Read the model definition and answer for the solid it produces. Units are mm, in the model's axes. A direction names the side the tool comes from. Coordinates: 2 decimals unless noted, no trailing zeros. Loops run counter-clockwise (first coordinate to the right, second up) from the corner with the lowest first, then second, coordinate; pieces in that order, holes last. Notation, with made-up numbers: (14.25, -39) -> (62.25, -39) arc R21 cw to (62.25, -6) -> close; hole circle Ø6 at (-21, 35). An arc over 180 degrees is marked (long way). Answer in a Markdown table with one row per item.
```python
from build123d import *

# Parameters (mm, degrees)
EXTRUSION1_DEPTH        = 5
ESQUISSE2_R             = 1.5
EXTRUSION2_DEPTH        = 3
CHANFREIN1_SIZE         = 0.2
ESQUISSE3_R             = 1.3
ENL_V_MAT_EXTRU_1_DEPTH = 3


with BuildPart() as part:
    # Esquisse1 → Extrusion1 (new body)
    with BuildSketch(Plane.XY):
        Polygon((1.443375673, 2.5), (-1.443375673, 2.5), (-2.886751346, 0), (-1.443375673, -2.5), (1.443375673, -2.5), (2.886751346, 0), align=None)
    extrude(amount=EXTRUSION1_DEPTH)

    # Esquisse2 → Extrusion2 (add)
    with BuildSketch(Plane(origin=(0, 0, 0), x_dir=(-1, 0, 0), z_dir=(0, 0, -1))):
        Circle(ESQUISSE2_R)
    extrude(amount=EXTRUSION2_DEPTH)

    # Chanfrein1
    chanfrein1_edges = [part.edges().sort_by_distance(p)[0] for p in [
        (1.5, 0, -3),
    ]]
    chamfer(chanfrein1_edges, length=CHANFREIN1_SIZE)

    # Esquisse3 → Enlèv. mat.-Extru.1 (cut)
    with BuildSketch(Plane.XY.offset(5)):
        Circle(ESQUISSE3_R)
    extrude(amount=-ENL_V_MAT_EXTRU_1_DEPTH, mode=Mode.SUBTRACT)

    # Esquisse4 → Enlèvement de matière-Révolution1 (revolve, cut)
    with BuildSketch(Plane(origin=(0, 0, 0), x_dir=(1, 0, 0), z_dir=(0, 1, 0)), mode=Mode.PRIVATE) as enl_vement_de_mati_re_r_volution1_sk:
        with BuildLine():
            Line((1.2, 0.617157288), (1.2, 0.2))
            ThreePointArc((1.2, 0.2), (1.258578644, 0.058578644), (1.4, 0))
            Line((1.4, 0), (1.804772915, 0))
            Line((1.804772915, 0), (1.804772915, 1.304772915))
            Line((1.804772915, 1.304772915), (1.258578644, 0.758578644))
            ThreePointArc((1.258578644, 0.758578644), (1.215224093, 0.693693974), (1.2, 0.617157288))
        make_face()
    revolve(enl_vement_de_mati_re_r_volution1_sk.sketch.rotate(Axis((0, 0, -4.374841009), (0, 0, 1)), 180), axis=Axis((0, 0, -4.374841009), (0, 0, 1)), mode=Mode.SUBTRACT)


solid = part.part
```
1. A cutting plane is placed at D-D on x = -1.95. Give the vertices of the cut face in (y, z).
A:
| item | result |
|---|---|
| outline | (-1.62, 0) -> (1.62, 0) -> (1.62, 5) -> (-1.62, 5) -> close |
2. A tool of negligible diameter and unlimited length cuts with its end or side. For faces 5 (the cylindrical face through (1.5, 0.07, -1.89)), 6 (the flat face through (2.175, 1.233, 2.465)), 7 (the cylindrical face through (-0.65, -1.01, -0.41)), from which of +Z, -Z, +X, -X, +Y, -Y can it reach the whole face along a straight path? Write none if from no direction.
A:
| item | result |
|---|---|
| face 5 | -Z |
| face 6 | +Z, -Z, +X, +Y |
| face 7 | none |
3. A cutting plane is placed at A-A on z = 1.75. Give the vertices of the cut face in (x, y).
A:
| item | result |
|---|---|
| outline | (-2.89, 0) -> (-1.44, -2.5) -> (1.44, -2.5) -> (2.89, 0) -> (1.44, 2.5) -> (-1.44, 2.5) -> close |
4. A cutting plane is placed at B-B on x = 0. Give the vertices of the cut face in (y, z), and give its area (3 significant figures).
A:
| item | result |
|---|---|
| outline | (-2.5, 0) -> (-1.4, 0) arc R0.2 cw to (-1.2, -0.2) -> (-1.2, -0.62) arc R0.2 cw to (-1.26, -0.76) -> (-1.5, -1) -> (-1.5, -2.8) -> (-1.3, -3) -> (1.3, -3) -> (1.5, -2.8) -> (1.5, -1) -> (1.26, -0.76) arc R0.2 cw to (1.2, -0.62) -> (1.2, -0.2) arc R0.2 cw to (1.4, 0) -> (2.5, 0) -> (2.5, 5) -> (1.3, 5) -> (1.3, 2) -> (-1.3, 2) -> (-1.3, 5) -> (-2.5, 5) -> close |
| area | 25.7 mm2 |
5. A cutting plane is placed at C-C on y = -2. Give the vertices of the cut face in (x, z).
A:
| item | result |
|---|---|
| outline | (-1.73, 0) -> (1.73, 0) -> (1.73, 5) -> (-1.73, 5) -> close |
6. The mould has two halves that part along X. Classify faces 1 (the cylindrical face through (-0.17, 1.29, 3.52)), 2 (the flat face through (1.2, 1.1, 0)), 3 (the flat face through (0, 0, 2)), 4 (the flat face through (-2.155, 1.267, 2.465)): pulls with the +X half, pulls with the -X half, needs draft (parallel to the pull), parting line crosses it, or undercut.
A:
| item | result |
|---|---|
| face 1 | undercut |
| face 2 | needs draft |
| face 3 | undercut |
| face 4 | pulls with the -X half |
7. Find the intervals of material crossed by probe 1 along Y at (x, z) = (0, 4.35); probe 2 along Z at (x, y) = (-1.6, 1.1); probe 3 along X at (y, z) = (0.05, -1.5), in increasing order.
A:
| item | result |
|---|---|
| probe 1 | y = -2.5 to -1.3, 1.3 to 2.5 |
| probe 2 | z = 0 to 5 |
| probe 3 | x = -1.5 to 1.5 |
8. Given pin 1 Ø0.8 at (x, y) = (0, 0.5) entering from +Z; pin 2 Ø1 at (x, z) = (1, -2) entering from +Y; pin 3 Ø3 at (x, y) = (-1, 0) entering from +Z, each flat-ended and moving along its own axis, determine where each tip first touches the part or whether it passes through.
A:
| item | result |
|---|---|
| pin 1 | stops at z = 2 |
| pin 2 | stops at y = 1.41 |
| pin 3 | stops at z = 5 |
